from build123d import *

# Parameters (mm, degrees)
F0_R     = 85.09
F0_R_2   = 78.74
F1_DEPTH = 6.35
F2_R     = 3.175
F3_DEPTH = 95.25


with BuildPart() as f1:
    # F0 (on Front) → F1 (new body)
    with BuildSketch(Plane.XZ):
        Circle(F0_R)
        Circle(F0_R_2, mode=Mode.SUBTRACT)
    extrude(amount=F1_DEPTH)

    # F2 (on Right) → F3 (join, symmetric)
    with BuildSketch(Plane.YZ):
        with Locations((-3.175, 0)):
            Circle(F2_R)
    extrude(amount=F3_DEPTH, both=True)


solid = f1.part
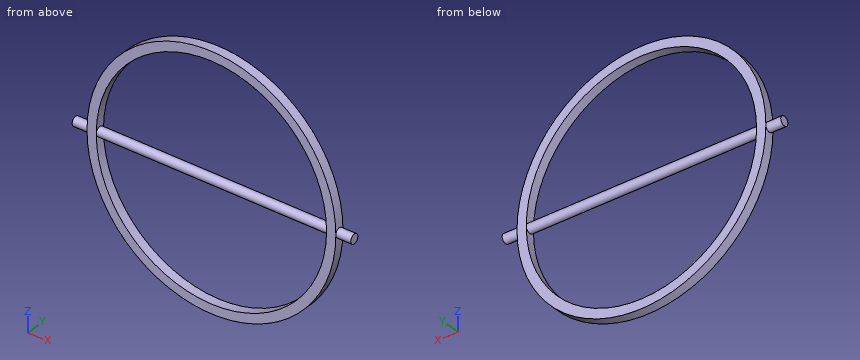
Verification items for the finished model (mm, model axes). Give positions to 0.01 mm unless a question says otherwise; leave off trailing zeros. Write each loop counter-clockwise with the first axis right and the second up, starting at its lowest first coordinate (ties: lowest second). Pieces come first, ordered by that corner, then holes.
(1) Material ranges on line 1 (Z direction, x = 44.5, y = -3); line 2 (Z direction, x = -61.5, y = -5.25); line 3 (X direction, y = -4.75, z = 16), recorded low to high.
(2) Gauge pin test, flat ends, axial feed: pin 1 (1.5 mm diameter, centred on y = -3.5, z = 19.5, fed in from +X); pin 2 (3 mm diameter, centred on y = -3.5, z = -7, fed in from -X). Record the tip position at first contact, or that the pin passes through.
(3) Cross-section at B-B (z = 72). Enter the section's corners in (x, y).
(4) Cross-section at D-D (z = -57). Enter the section's corners in (x, y), plus the area to 3 significant figures.
(5) Cross-section at A-A (x = 0). Enter the section's corners in (y, z) (3 decimals), plus the area to 3 significant figures.
Worked out:
1. line 1: z = -72.53 to -64.96, -3.17 to 3.17, 64.96 to 72.53
1. line 2: z = -58.81 to -49.17, -2.4 to 2.4, 49.17 to 58.81
1. line 3: x = -83.57 to -77.1, 77.1 to 83.57
2. pin 1: stops at x = 83
2. pin 2: stops at x = -84.91
3. outline: (-45.35, -6.35) - (-31.87, -6.35) - (-31.87, 0) - (-45.35, 0) - close; (31.87, -6.35) - (45.35, -6.35) - (45.35, 0) - (31.87, 0) - close
4. outline: (-63.18, -6.35) - (-54.32, -6.35) - (-54.32, 0) - (-63.18, 0) - close; (54.32, -6.35) - (63.18, -6.35) - (63.18, 0) - (54.32, 0) - close
4. area: 112 mm2
5. outline: (-6.35, -85.09) - (0, -85.09) - (0, -78.74) - (-6.35, -78.74) - close; circle Ø6.35 at (-3.175, 0); (-6.35, 78.74) - (0, 78.74) - (0, 85.09) - (-6.35, 85.09) - close
5. area: 112 mm2
